Verification items for the finished model (mm, model axes). Give positions to 0.01 mm unless a question says otherwise; leave off trailing zeros. Order: outer loops, then holes, each group sorted by start corner. A loop starts at its lowest first (then second) coordinate and runs counter-clockwise, first axis right, second up. Notation, with made-up numbers: (52, 5.25) -> (70, 5.25) arc R20 ccw to (70, 14.25) -> close; hole circle Ø3 at (69, -26.75). An arc over 180 degrees is marked (long way). Write each question's results on one line, items separated by ' | '. Start each with the question number.
1. Cross-section at A-A, the plane x = 0. Enter the section's corners in (y, z) (3 decimals).
2. Cross-section at B-B, the plane z = 3.75. Enter the section's corners in (x, y) (3 decimals), then the cut area to 3 significant figures.
3. Mould release check, pull along X, two halves, no side actions. Record for faces 1 (the face through (-17.99, -1.26, 3.15)), 2 (the face through (13.785, 7.873, 3.148)), 3 (the face through (4, -12, 6.35)), 4 (the face through (10.083, -14.947, 3.148)): +X half, -X half, draft (parallel to the pull), parting line (faces both ways), or undercut.
4. Depth check by flat-ended pin: pin 1 Ø8 at (x, y) = (9.5, -15.5) entering from -Z; pin 2 Ø2 at (x, z) = (13, 5) entering from -Y. Enter the tip coordinate at first touch or a pass-through.
5. Material ranges on L1, parallel to Y at x = 0, z = 4.5 (3 decimals); L2, parallel to Y at x = -8.5, z = 2.75; L3, parallel to Y at x = -7, z = 4.75, recorded low to high. Write a range as from..to.
from build123d import *

# Parameters (mm, degrees)
F0_R     = 11.0363
F1_DEPTH = 6.35
F2_SIZE  = 1.27


# Not quite as in the source:
# - a feature names something its author has since deleted; it is built from what else it names


with BuildPart() as f1:
    # F0 (on Top) → F1 (new body)
    with BuildSketch(Plane.XY):
        with BuildLine():
            ThreePointArc((13.7481534459, -7.9374997215), (15.334072534, -4.1087521857), (15.875, 0))
            ThreePointArc((15.875, 0), (15.8042735617, 1.4968507561), (15.592724449, 2.9803639471))
            ThreePointArc((15.592724449, 2.9803639471), (13.7481532851, 7.9375), (10.3774331152, 12.0135135135))
            ThreePointArc((10.3774331152, 12.0135135135), (5.5362937901, 14.8783425176), (-1.09e-08, 15.875))
            ThreePointArc((-1.09e-08, 15.875), (-5.5362938003, 14.8783425138), (-10.3774331152, 12.0135135135))
            ThreePointArc((-10.3774331152, 12.0135135135), (-13.7481532851, 7.9375), (-15.592724449, 2.9803639471))
            ThreePointArc((-15.592724449, 2.9803639471), (-15.6531695071, -2.6446000421), (-13.7481534335, -7.9374997429))
            ThreePointArc((-13.7481534335, -7.9374997429), (-10.1168758016, -12.2337422327), (-5.2152913338, -14.9938774606))
            ThreePointArc((-5.2152913338, -14.9938774606), (0, -15.875), (5.2152913338, -14.9938774606))
            ThreePointArc((5.2152913338, -14.9938774606), (10.1168758111, -12.2337422248), (13.7481534459, -7.9374997215))
        make_face()
        Circle(F0_R, mode=Mode.SUBTRACT)
        with BuildLine():
            ThreePointArc((15.592724449, 2.9803639471), (15.8042735617, 1.4968507561), (15.875, 0))
            ThreePointArc((15.875, 0), (15.334072534, -4.1087521857), (13.7481534459, -7.9374997215))
            ThreePointArc((13.7481534459, -7.9374997215), (17.4968931029, -4.3051053849), (22.5971491052, -3.1939229768))
            ThreePointArc((22.5971491052, -3.1939229768), (18.038469294, -1.3052898819), (15.592724449, 2.9803639471))
        make_face()
        with BuildLine():
            ThreePointArc((14.0645929883, -17.9727436898), (12.4767771707, -13.0002009006), (13.7481534459, -7.9374997215))
            ThreePointArc((13.7481534459, -7.9374997215), (10.1168758111, -12.2337422248), (5.2152913338, -14.9938774606))
            ThreePointArc((5.2152913338, -14.9938774606), (10.149648844, -14.9691277131), (14.0645929883, -17.9727436898))
        make_face()
        with BuildLine():
            ThreePointArc((22.5971491052, -3.1939229768), (17.4968931029, -4.3051053849), (13.7481534459, -7.9374997215))
            ThreePointArc((13.7481534459, -7.9374997215), (12.4767771707, -13.0002009006), (14.0645929883, -17.9727436898))
            ThreePointArc((14.0645929883, -17.9727436898), (24.751043908, -21.81817506), (31.5220452561, -12.7))
            ThreePointArc((31.5220452561, -12.7), (28.9411655806, -6.1804280878), (22.5971491052, -3.1939229768))
        make_face()
        with BuildLine():
            ThreePointArc((-1.09e-08, 15.875), (5.5362937901, 14.8783425176), (10.3774331152, 12.0135135135))
            ThreePointArc((10.3774331152, 12.0135135135), (7.88882045, 16.274417595), (8.5325561169, 21.1666666667))
            ThreePointArc((8.5325561169, 21.1666666667), (5.0201157809, 17.3053065193), (-1.09e-08, 15.875))
        make_face()
        with BuildLine():
            ThreePointArc((-10.3774331152, 12.0135135135), (-5.5362938003, 14.8783425138), (-1.09e-08, 15.875))
            ThreePointArc((-1.09e-08, 15.875), (-5.0201157901, 17.305306525), (-8.5325561169, 21.1666666667))
            ThreePointArc((-8.5325561169, 21.1666666667), (-7.88882045, 16.274417595), (-10.3774331152, 12.0135135135))
        make_face()
        with BuildLine():
            ThreePointArc((-8.5325561169, 21.1666666667), (-5.0201157901, 17.305306525), (-1.09e-08, 15.875))
            ThreePointArc((-1.09e-08, 15.875), (5.0201157809, 17.3053065193), (8.5325561169, 21.1666666667))
            ThreePointArc((8.5325561169, 21.1666666667), (9.2735705641, 23.2259452645), (9.525, 25.4))
            ThreePointArc((9.525, 25.4), (-2.1740547355, 34.6735705641), (-8.5325561169, 21.1666666667))
        make_face()
        with BuildLine():
            ThreePointArc((-14.0645929883, -17.9727436898), (-10.149648844, -14.9691277131), (-5.2152913338, -14.9938774606))
            ThreePointArc((-5.2152913338, -14.9938774606), (-10.1168758016, -12.2337422327), (-13.7481534335, -7.9374997429))
            ThreePointArc((-13.7481534335, -7.9374997429), (-12.7966017991, -10.234748452), (-12.4720452561, -12.7))
            ThreePointArc((-12.4720452561, -12.7), (-12.8788701961, -15.4539986519), (-14.0645929883, -17.9727436898))
        make_face()
        with BuildLine():
            ThreePointArc((-22.5971491052, -3.1939229768), (-17.496893092, -4.3051053908), (-13.7481534335, -7.9374997429))
            ThreePointArc((-13.7481534335, -7.9374997429), (-15.6531695071, -2.6446000421), (-15.592724449, 2.9803639471))
            ThreePointArc((-15.592724449, 2.9803639471), (-18.038469294, -1.3052898819), (-22.5971491052, -3.1939229768))
        make_face()
        with BuildLine():
            ThreePointArc((-12.4720452561, -12.7), (-12.7966017991, -10.234748452), (-13.7481534335, -7.9374997429))
            ThreePointArc((-13.7481534335, -7.9374997429), (-17.496893092, -4.3051053908), (-22.5971491052, -3.1939229768))
            ThreePointArc((-22.5971491052, -3.1939229768), (-30.2459372272, -17.4625), (-14.0645929883, -17.9727436898))
            ThreePointArc((-14.0645929883, -17.9727436898), (-12.8788701961, -15.4539986519), (-12.4720452561, -12.7))
        make_face()
    extrude(amount=F1_DEPTH)

    # F2
    f2_edges = [f1.edges().sort_by_distance(p)[0] for p in [
        (13.748153, 7.9375, 0),
        (7.88882, 16.274418, 0),
        (0, 34.925, 0),
        (-7.88882, 16.274418, 0),
        (-13.748153, 7.9375, 0),
        (-18.038469, -1.30529, 0),
        (-30.245937, -17.4625, 0),
        (-10.149649, -14.969128, 0),
        (0, -15.875, 0),
        (10.149649, -14.969128, 0),
        (30.245937, -17.4625, 0),
        (18.038469, -1.30529, 0),
        (-11.0363, 0, 0),
        (13.748153, 7.9375, 6.35),
        (7.88882, 16.274418, 6.35),
        (0, 34.925, 6.35),
        (-7.88882, 16.274418, 6.35),
        (-13.748153, 7.9375, 6.35),
        (-18.038469, -1.30529, 6.35),
        (-30.245937, -17.4625, 6.35),
        (-10.149649, -14.969128, 6.35),
        (0, -15.875, 6.35),
        (10.149649, -14.969128, 6.35),
        (30.245937, -17.4625, 6.35),
        (18.038469, -1.30529, 6.35),
        (-11.0363, 0, 6.35),
    ]]
    chamfer(f2_edges, length=F2_SIZE)


solid = f1.part
Results below:
1) outline: (-15.875, 1.27) -> (-14.605, 0) -> (-12.306, 0) -> (-11.036, 1.27) -> (-11.036, 5.08) -> (-12.306, 6.35) -> (-14.605, 6.35) -> (-15.875, 5.08) -> close; (11.036, 1.27) -> (12.306, 0) -> (33.655, 0) -> (34.925, 1.27) -> (34.925, 5.08) -> (33.655, 6.35) -> (12.306, 6.35) -> (11.036, 5.08) -> close
2) outline: (-22.597, -3.194) arc R9.525 ccw (long way) to (-14.065, -17.973) arc R7.62 cw to (-5.215, -14.994) arc R15.875 ccw to (5.215, -14.994) arc R7.62 cw to (14.065, -17.973) arc R9.525 ccw (long way) to (22.597, -3.194) arc R7.62 cw to (15.593, 2.98) arc R15.875 ccw to (10.377, 12.014) arc R7.62 cw to (8.533, 21.167) arc R9.525 ccw (long way) to (-8.533, 21.167) arc R7.62 cw to (-10.377, 12.014) arc R15.875 ccw to (-15.593, 2.98) arc R7.62 cw to start; hole circle Ø22.073 at (0, 0) | area: 1,360 mm²
3) face 1: -X half | face 2: +X half | face 3: draft | face 4: undercut
4) pin 1: stops at z = 0 | pin 2: stops at y = -17.88
5) L1: y = -15.875..-11.036, 11.036..34.925 | L2: y = -14.61..-7.04, 7.04..14.46, 21.1..29.7 | L3: y = -14.6..-8.53, 8.53..31.86
